```python
from build123d import *

# Parameters (mm, degrees)
BOSS_EXTRUDE3_DEPTH = 1.6
CUT_EXTRUDE3_DEPTH  = 1249.077106674


with BuildPart() as part:
    # Sketch5 → Boss-Extrude3 (new body)
    with BuildSketch(Plane(origin=(0, 0, 0), x_dir=(1, 0, 0), z_dir=(0, 1, 0))):
        Polygon((0, 0), (628, 0), (628, -230.8), (604.512792249, -826.1), (509.77, -1078.56845133), (118.23, -1078.56845133), (23.487207751, -826.1), (0, -230.8), align=None)
    extrude(amount=BOSS_EXTRUDE3_DEPTH)

    # Sketch6 → Cut-Extrude3 (cut, through all)
    with BuildSketch(Plane(origin=(0, 1.6, 0), x_dir=(1, 0, 0), z_dir=(0, 1, 0))):
        Polygon((23.487207751, -826.1), (604.512792249, -826.1), (509.77, -1078.56845133), (118.23, -1078.56845133), align=None)
    extrude(amount=-CUT_EXTRUDE3_DEPTH, mode=Mode.SUBTRACT)


solid = part.part
```
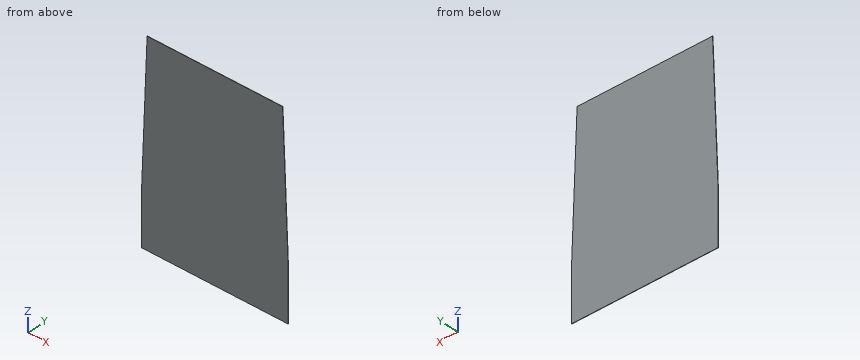
Build history of the part. All positions in model axes, mm. Coordinates: 2 decimals unless noted, no trailing zeros. Write each loop counter-clockwise with the first axis right and the second up, starting at its lowest first coordinate (ties: lowest second). Pieces come first, ordered by that corner, then holes.
1. Band-saw the part on B-B, the plane z = 372. Give the cut face in (x, y).
Answer block:
outline: (5.57, 0) - (622.43, 0) - (622.43, 1.6) - (5.57, 1.6) - close
2. Band-saw the part on C-C, the plane z = 667. Give the cut face in (x, y), and give its area (3 significant figures).
Answer block:
outline: (17.21, 0) - (610.79, 0) - (610.79, 1.6) - (17.21, 1.6) - close
area: 950 mm2
3. Band-saw the part on A-A, the plane y = 0.95. Give the cut face in (x, z).
Answer block:
outline: (0, 0) - (628, 0) - (628, 230.8) - (604.51, 826.1) - (23.49, 826.1) - (0, 230.8) - close
4. Drill centre lines: probe 1 along X at (y, z) = (1.25, 424.5); probe 2 along X at (y, z) = (1.1, 706). Where is each one in solid material? Low to high.
Answer block:
probe 1: x = 7.64 to 620.36
probe 2: x = 18.75 to 609.25
